from build123d import *

# Parameters (mm, degrees)
F1_DEPTH = 3
F2_D     = 3.5
F3_W     = 4
F3_H     = 9
F4_DEPTH = 14
F5_W     = 4
F5_H     = 9
F6_DEPTH = 3
F7_R     = 5


with BuildPart() as f1:
    # F0 (on Front) → F1 (new body)
    with BuildSketch(Plane.XZ):
        Polygon((-9, 9), (-9, 0), (9, 0), (9, 9), (9, 18), (-9, 18), align=None)
    extrude(amount=F1_DEPTH)

    # F2 (through all)
    with Locations(Plane(origin=(0, 0, 0), x_dir=(1, 0, 0), z_dir=(0, 1, 0))):
        with Locations((-5, -13), (5, -13)):
            Hole(F2_D / 2)

    # F3 (on face) → F4 (join)
    with BuildSketch(Plane.XZ):
        with Locations((0, 4.5)):
            Rectangle(F3_W, F3_H)
    extrude(amount=-F4_DEPTH)

    # F5 (on face) → F6 (join)
    with BuildSketch(Plane(origin=(0, 14, 0), x_dir=(-1, 0, 0), z_dir=(0, 1, 0))):
        Polygon((9, 0), (9, 18), (-2, 18), (-2, 9), (2, 9), (2, 0), align=None)
        with BuildLine():
            ThreePointArc((5.5, 16.25), (6.7374368671, 15.7374368671), (7.25, 14.5))
            Line((7.25, 14.5), (7.25, 3.5))
            ThreePointArc((7.25, 3.5), (6.7374368671, 2.2625631329), (5.5, 1.75))
            ThreePointArc((5.5, 1.75), (4.2625631329, 2.2625631329), (3.75, 3.5))
            Line((3.75, 3.5), (3.75, 14.5))
            ThreePointArc((3.75, 14.5), (4.2625631329, 15.7374368671), (5.5, 16.25))
        make_face(mode=Mode.SUBTRACT)
        with Locations((0, 4.5)):
            Rectangle(F5_W, F5_H)
    extrude(amount=F6_DEPTH)

    # F7
    f7_edges = [f1.edges().sort_by_distance(p)[0] for p in [
        (9, -1.5, 18),
        (-9, -1.5, 18),
        (2, 15.5, 18),
    ]]
    fillet(f7_edges, radius=F7_R)


solid = f1.part
Here's how the part is built. I have some questions about the finished solid (model axes, mm). A direction names the side the tool comes from. Coordinates: 2 decimals unless noted, no trailing zeros. Write each loop counter-clockwise with the first axis right and the second up, starting at its lowest first coordinate (ties: lowest second). Pieces come first, ordered by that corner, then holes. Notation, with made-up numbers: (-6, 54.25) - (30, 54.25) arc R11 ccw to (30, 71.25) - close; hole circle Ø6 at (44.25, 31.5). An arc over 180 degrees is marked (long way). Use one line per item in the form item = value.
1) I'm going to push flat-ended pins straight in: P1, Ø3.5, axis at y = 15, z = 9.5, coming from the +X side; P2, Ø2.5, axis at y = 3.5, z = 2.5, coming from the -X side; P3, Ø2, axis at x = 5, z = 13, coming from the +Y side; P4, Ø3, axis at x = 0.5, y = 8, coming from the +Z side. Where does each tip first touch, or does it pass through?
Solved:
P1 = 2
P2 = -2
P3 = through
P4 = 9
2) Suppose I cut it at B-B, the plane x = -5. Write out the boundary of the cut face in (y, z).
Solved:
outline = (-3, 0) - (0, 0) - (0, 11.25) - (-3, 11.25) - close; (-3, 14.75) - (0, 14.75) - (0, 17.9) - (-3, 17.9) - close; (14, 0) - (17, 0) - (17, 1.82) - (14, 1.82) - close; (14, 16.18) - (17, 16.18) - (17, 18) - (14, 18) - close
3) Thinking about a two-plate mould opening in Z: for faces 4 (the cylindrical face through (8, -2, 16)), 5 (the cylindrical face through (-4.772, -1.521, 11.265)), 6 (the flat face through (-1, 6, 0)), which applies, released by +Z, released by -Z, zero draft, split by the parting line, or undercut?
Solved:
face_4 = released by +Z
face_5 = undercut
face_6 = released by -Z
4) Suppose I cut it at D-D, the plane y = -0.75. Write out the boundary of the cut face in (x, z), plus the area to 3 significant figures.
Solved:
outline = (-9, 0) - (9, 0) - (9, 13) arc R5 ccw to (4, 18) - (-4, 18) arc R5 ccw to (-9, 13) - close; hole circle Ø3.5 at (-5, 13); hole circle Ø3.5 at (5, 13)
area = 294 mm2
5) Suppose I cut it at A-A, the plane z = 4. Write out the boundary of the cut face in (x, y), plus the area to 4 significant figures.
Solved:
outline = (-9, -3) - (9, -3) - (9, 0) - (2, 0) - (2, 17) - (-3.75, 17) - (-3.75, 14) - (-2, 14) - (-2, 0) - (-9, 0) - close; (-9, 14) - (-7.25, 14) - (-7.25, 17) - (-9, 17) - close
area = 132.5 mm2
6) On a 3-axis mill with a long thin cutter (end or side, diameter ignored), from which of +Z, -Z, +X, -X, +Y, -Y can I reach the whole of each face in a straight line? I mean faces 1 (the flat face through (-3, 14, 9)), 2 (the cylindrical face through (1, 16, 16)), 3 (the flat face through (0, 7, 9)). Say none if no direction works.
Solved:
face_1 = +Z, -X
face_2 = +Z, +X, +Y
face_3 = +Z, +X, -X
7) I need wall thicknesses on line 1 (X direction, y = -1.35, z = 13); line 2 (Y direction, x = -5.75, z = 1); line 3 (X direction, y = 16, z = 8.25). Which ranges of each line are inside material? Lowest first, please.
Solved:
line_1 = -9 to -6.75, -3.25 to 3.25, 6.75 to 9
line_2 = -3 to 0, 14 to 17
line_3 = -9 to -7.25, -3.75 to 2
8) Suppose I cut it at C-C, the plane z = 9.75. Write out the boundary of the cut face in (x, y), plus the area to 3 significant figures.
Solved:
outline = (-9, -3) - (9, -3) - (9, 0) - (-9, 0) - close; (-9, 14) - (-7.25, 14) - (-7.25, 17) - (-9, 17) - close; (-3.75, 14) - (2, 14) - (2, 17) - (-3.75, 17) - close
area = 76.5 mm2
